Autodesk Inventor part; units mm, degrees
ref_plane "YZ Plane" through (0, 0, 0) normal (1, 0, 0) x (0, 1, 0)
ref_plane "XZ Plane" through (0, 0, 0) normal (0, 1, 0) x (-1, 0, 0)
ref_plane "XY Plane" through (0, 0, 0) normal (0, 0, 1) x (1, 0, 0)
sketch "Skizze1" plane through (0, 0, 0) normal (1, 0, 0) x (0, 1, 0)
  line L0 (0, 0) -> (0, -60)
  line L1 (0, 0) -> (10, 0)
  line L2 (10, 0) -> (10, -60)
  line L3 (10, -60) -> (0, -60)
  line L4 (10, -60) -> (10, -60)
  line L5 (10, -60) -> (10, -8.2526)
  line L6 (10, -8.2526) -> (10, 0)
  line L7 (0, -30) -> (87.5, -30)
  circle A0 centre (87.5, -30) radius 42.5
  line L8 (10, 0) -> (20, 0)
  line L9 (10, -60) -> (20.0931, -60)
  line L10 (59.9602, 2.3699) -> (43.8038, -11.3757)
  line L11 (20, 0) -> (32.2885, -11.3757)
  line L12 (32.2885, -11.3757) -> (43.8038, -11.3757)
  line L13 (20.0931, -60) -> (32.2885, -48.6243)
  line L14 (32.2885, -48.6243) -> (43.8038, -48.6243)
  line L15 (43.8038, -48.6243) -> (59.9602, -62.3699)
  line L16 (38.0462, -11.3757) -> (38.0462, -48.6243)
  line L17 (130, -30) -> (87.5, -30)
  dimension "d0" = 20
  dimension "d1" = 60
  dimension "d2" = 85
  dimension "d4" = 260
  dimension "d5" = 40
revolve "Umdrehung1" add sketch "Skizze1" angle 360 about axis through (0, 0, 0) along (0, 0, -1) contours L8 L11 L12 L16 L7 L2 | L7 L16 L14 L13 L9 L2 | L16 L12 L10 A0 L7 | L7 A0 L15 L14 L16 | A0 L17 L7 | L7 L17 A0
properties part number "Wheel"
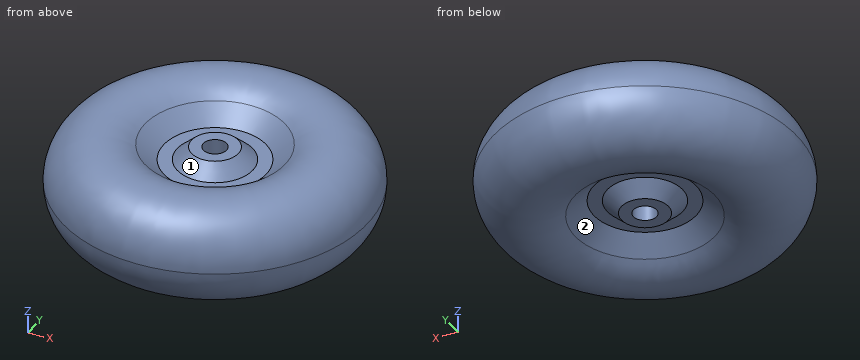
Verification items for the finished model (mm, model axes). Face numbers are marked on the shaded views. Coordinates: 2 decimals unless noted, no trailing zeros. Write each loop counter-clockwise with the first axis right and the second up, starting at its lowest first coordinate (ties: lowest second). Pieces come first, ordered by that corner, then holes. Notation, with made-up numbers: M -30,8.25 L -23,8.25 A25 ccw -23,30.25 Z; hole C 59.25,-13 d5. An arc over 180 degrees is marked long. Use a Markdown table: item, result.
Q1. Thickness scan on line 1 (Y direction, x = -46.5, z = -0.5); line 2 (Z direction, x = -11.5, y = -32.5); line 3 (X direction, y = 0, z = -19.5). Record the ranges inside material, lowest first.
Reply:
| item | result |
|---|---|
| line 1 | y = -108.55 to -32.25, 32.25 to 108.55 |
| line 2 | z = -48.62 to -11.38 |
| line 3 | x = -128.68 to -10, 10 to 128.68 |
Q2. Sectioned sample at A-A, the plane y = 0. Record the boundary of the cut face in (x, z).
Reply:
| item | result |
|---|---|
| outline | M -59.96,-62.37 L -43.8,-48.62 L -32.29,-48.62 L -20.09,-60 L -10,-60 L -10,0 L -20,0 L -32.29,-11.38 L -43.8,-11.38 L -59.96,2.37 A42.5 ccw long Z; M 10,-60 L 20.09,-60 L 32.29,-48.62 L 43.8,-48.62 L 59.96,-62.37 A42.5 ccw long 59.96,2.37 L 43.8,-11.38 L 32.29,-11.38 L 20,0 L 10,0 Z |
Q3. Sectioned sample at C-C, the plane z = -17. Record the boundary of the cut face in (x, y).
Reply:
| item | result |
|---|---|
| outline | C 0,0 d255.93; hole C 0,0 d20 |
Q4. Draft check along X on the marked faces 1 and 2. Enter one of: +X half, -X half, draft (parallel to the pull), parting line (faces both ways), or undercut.
Reply:
| item | result |
|---|---|
| face 1 | undercut |
| face 2 | undercut |
Q5. Go/stop test with flat-tipped pins: P1, Ø1, axis at y = 28.5, z = -27.5, coming from the +X side; P2, Ø2, axis at x = 1.5, z = -9.5, coming from the -Y side; P3, Ø2, axis at x = -81, y = 93.5, coming from the +Z side. Record where each tip stops, or that it passes through.
Reply:
| item | result |
|---|---|
| P1 | stops at x = 126.88 |
| P2 | stops at y = -125.25 |
| P3 | stops at z = -6.19 |
Q6. Sectioned sample at D-D, the plane z = -44.5. Record the boundary of the cut face in (x, y).
Reply:
| item | result |
|---|---|
| outline | C 0,0 d254.9; hole C 0,0 d20 |
